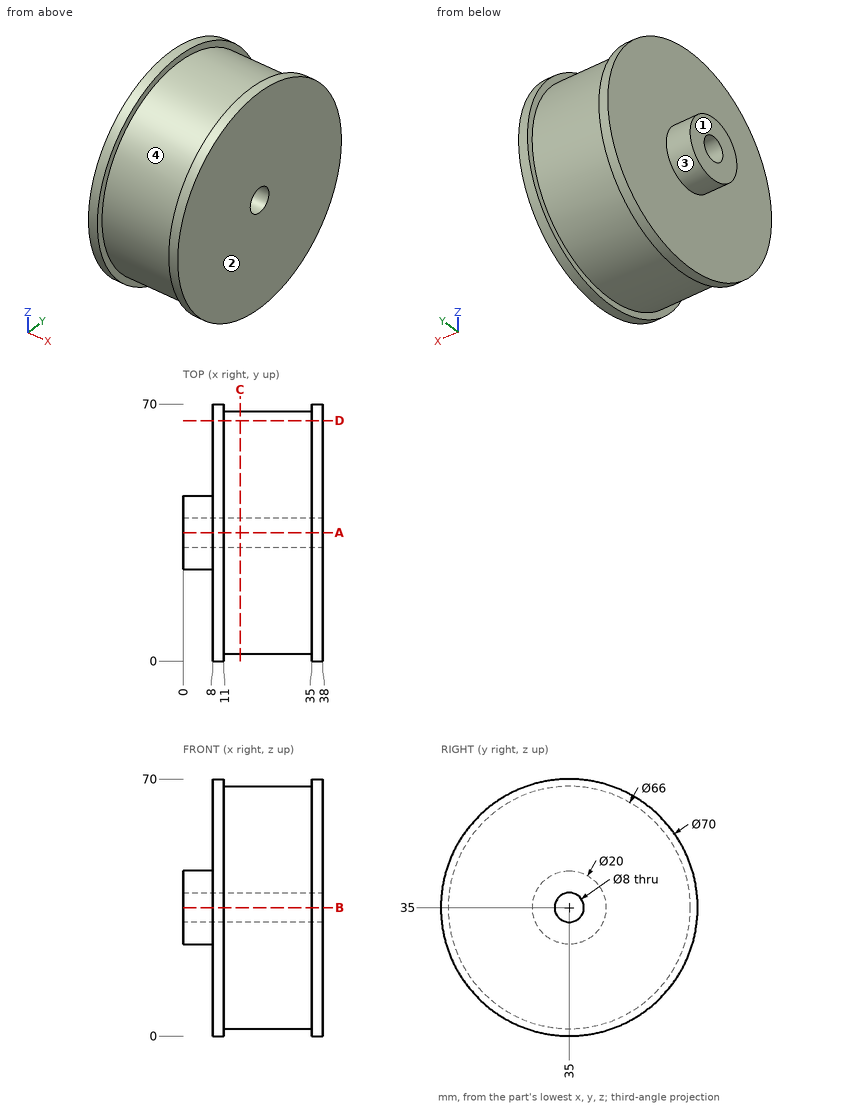
Could you check a few things on this drawing? It's one solid part, dimensions in mm from its lowest x, y, z. Coordinates: 2 decimals unless noted, no trailing zeros. Order: outer loops, then holes, each group sorted by start corner. A loop starts at its lowest first (then second) coordinate and runs counter-clockwise, first axis right, second up.
1. Thinking about a two-plate mould opening in X: for the marked faces 1, 2, 3 and 4, which applies, +X half, -X half, draft (parallel to the pull), parting line (faces both ways), or undercut?
2. If we section it at A-A (y = 35): Please give me the cut outline in (x, z), then the cut area to 3 significant figures.
3. If we section it at C-C (x = 15.5): Please give me the cut outline in (y, z).
4. I'm going to push flat-ended pins straight in: pin 1 (5 mm diameter, centred on x = 15.5, z = 12, fed in from -Y); pin 2 (1 mm diameter, centred on x = 25, z = 17.5, fed in from -Y); pin 3 (4 mm diameter, centred on x = 31.5, y = 15, fed in from +Z). Where does each tip first touch, or does it pass through?
5. I need wall thicknesses on line 1 (X direction, y = 28.5, z = 4.5); line 2 (X direction, y = 5, z = 18.5); line 3 (Z direction, x = 28.5, y = 36). Which ranges of each line are inside material? Lowest first, please.
6. If we section it at D-D (y = 65.5): Please give me the cut outline in (x, z), then the cut area to 3 significant figures.
Entries:
1. face 1: -X half
1. face 2: +X half
1. face 3: draft
1. face 4: undercut
2. outline: (0, 25) - (8, 25) - (8, 0) - (11, 0) - (11, 2) - (35, 2) - (35, 0) - (38, 0) - (38, 31) - (0, 31) - close; (0, 39) - (38, 39) - (38, 70) - (35, 70) - (35, 68) - (11, 68) - (11, 70) - (8, 70) - (8, 45) - (0, 45) - close
2. area: 1,860 mm2
3. outline: circle Ø66 at (35, 35); hole circle Ø8 at (35, 35)
4. pin 1: stops at y = 9.14
4. pin 2: stops at y = 6.72
4. pin 3: stops at z = 62.66
5. line 1: x = 8 to 38
5. line 2: x = 8 to 11, 35 to 38
5. line 3: z = 2.02 to 31.13, 38.87 to 67.98
6. outline: (8, 17.83) - (11, 17.83) - (11, 22.4) - (35, 22.4) - (35, 17.83) - (38, 17.83) - (38, 52.17) - (35, 52.17) - (35, 47.6) - (11, 47.6) - (11, 52.17) - (8, 52.17) - close
6. area: 811 mm2
